Here's how the part is built. I have some questions about the finished solid (model axes, mm). Coordinates: 2 decimals unless noted, no trailing zeros. Write each loop counter-clockwise with the first axis right and the second up, starting at its lowest first coordinate (ties: lowest second). Pieces come first, ordered by that corner, then holes. Notation, with made-up numbers: M 62,-11 L 67,-11 A21 ccw 67,-4 Z; hole C -31,89.5 d7. An arc over 180 degrees is marked long. Write each question's results on one line, items separated by ' | '. Start each with the question number.
from build123d import *

# Parameters (mm, degrees)
F1_DEPTH = 3


with BuildPart() as f1:
    # F0 (on Top) → F1 (new body)
    with BuildSketch(Plane.XY):
        with BuildLine():
            Line((0, 0), (-18.5, 0))
            ThreePointArc((-18.5, 0), (-19.892913, -0.564802), (-20.499106, -1.940207))
            ThreePointArc((-20.499106, -1.940207), (-18.801318, -14.903789), (-13.108843, -26.67378))
            ThreePointArc((-13.108843, -26.67378), (0, -33.5), (13.108843, -26.67378))
            ThreePointArc((13.108843, -26.67378), (18.801318, -14.903789), (20.499106, -1.940207))
            ThreePointArc((20.499106, -1.940207), (19.892913, -0.564802), (18.5, 0))
            Line((18.5, 0), (0, 0))
        make_face()
    extrude(amount=F1_DEPTH)


solid = f1.part
1) I want a section at A-A, the plane z = 0.5. Write out the boundary of the cut face in (x, y).
2) For pin 1 Ø1.5 at (y, z) = (-13.5, 0.5) entering from +X, with a flat end and sliding along its axis, tell me the tip position at first contact or that it passes through.
3) I want a section at C-C, the plane x = -15.5. Write out the boundary of the cut face in (y, z), then the cut area to 3 significant figures.
4) Please list where these lines run through material, in increasing order: line 1 (X direction, y = -2, z = 2); line 2 (X direction, y = -29.5, z = 0.6); line 3 (Y direction, x = -12.5, z = 0.9). Write a range as [from, to].
5) I want a section at B-B, the plane y = -19. Write out the boundary of the cut face in (x, z).
Output:
1) outline: M -20.5,-1.94 A41 ccw -13.11,-26.67 A16 ccw 13.11,-26.67 A41 ccw 20.5,-1.94 A2 ccw 18.5,0 L -18.5,0 A2 ccw Z
2) pin 1: stops at x = 19.38
3) outline: M -22.82,0 L 0,0 L 0,3 L -22.82,3 Z | area: 68.5 mm2
4) line 1: x = [-20.5, 20.5] | line 2: x = [-10.58, 10.58] | line 3: y = [-27.49, 0]
5) outline: M -17.34,0 L 17.34,0 L 17.34,3 L -17.34,3 Z
